from build123d import *

# Parameters (mm, degrees)
SKETCH_R          = 8.35
SKETCH_R_2        = 3.95
PAD_DEPTH         = 219
SKETCH001_R       = 1.5
POCKET_DEPTH      = 100
POCKET_DEPTH_BACK = -100


with BuildPart() as part:
    # Sketch → Pad (new body)
    with BuildSketch(Plane.XY):
        Circle(SKETCH_R)
        Circle(SKETCH_R_2, mode=Mode.SUBTRACT)
    extrude(amount=PAD_DEPTH)

    # Sketch001 → Pocket (cut, two sides)
    with BuildSketch(Plane.XZ) as pocket_sk:
        with Locations((0, 109.5)):
            Circle(SKETCH001_R)
        with Locations((0, 189)):
            Circle(SKETCH001_R)
        with Locations((0, 30)):
            Circle(SKETCH001_R)
    extrude(amount=-POCKET_DEPTH, mode=Mode.SUBTRACT)
    extrude(pocket_sk.sketch, amount=-POCKET_DEPTH_BACK, mode=Mode.SUBTRACT)


solid = part.part
For this review, take the finished solid that the model builds, in its own axes (mm). Give positions to 0.01 mm unless a question says otherwise; leave off trailing zeros. Order: outer loops, then holes, each group sorted by start corner. A loop starts at its lowest first (then second) coordinate and runs counter-clockwise, first axis right, second up. Notation, with made-up numbers: (73.5, 39.5) - (90.5, 39.5) arc R15 ccw to (90.5, 64.5) - close; hole circle Ø4 at (-13.75, -23). An arc over 180 degrees is marked (long way). Answer as a JSON object with one key per item and string values. Group by question number.
Item 1: Take a section at A-A on y = 0. Give the boundary of the cut face in (x, z), and give its area (3 significant figures).
Item 2: Take a section at C-C on x = -6. Give the boundary of the cut face in (y, z).
Item 3: Wall thickness on line 1 along Z through (x, y) = (0, -6.35); line 2 along Z through (x, y) = (1, -5.25); line 3 along Y through (x, z) = (-1, 147): over which ranges is each line inside the solid? List them lowest first.
Item 4: Clearance check with flat-ended pins moving along their axes: pin 1 Ø1 at (x, z) = (-1.5, 77.5) entering from -Y; pin 2 Ø6 at (y, z) = (-6.5, 49.5) entering from -X; pin 3 Ø1 at (y, z) = (-6.5, 31.5) entering from +X. State where each tip first meets the part, or that it passes through.
Item 5: Draft analysis for pull direction X (two halves, no side actions). For faces 1 (the cylindrical face through (7.964, 2.508, 107.967)), 2 (the cylindrical face through (-3.135, -2.404, 107.967)), 3 (the flat face through (4, -2, 219)), state which applies: pulls with the +X half, pulls with the -X half, needs draft (parallel to the pull), parting line crosses it, or undercut.
Item 6: Take a section at B-B on z = 145. Give the boundary of the cut face in (x, y).
Reported:
{
 "1": {"outline": "(-8.35, 0) - (-3.95, 0) - (-3.95, 219) - (-8.35, 219) - close; (3.95, 0) - (8.35, 0) - (8.35, 219) - (3.95, 219) - close", "area": "1,930 mm^2"},
 "2": {"outline": "(-5.81, 0) - (5.81, 0) - (5.81, 219) - (-5.81, 219) - close"},
 "3": {"line 1": "0 to 28.5, 31.5 to 108, 111 to 187.5, 190.5 to 219", "line 2": "0 to 28.88, 31.12 to 108.38, 110.62 to 187.88, 190.12 to 219", "line 3": "-8.29 to -3.82, 3.82 to 8.29"},
 "4": {"pin 1": "y = -8.29", "pin 2": "x = -7.58", "pin 3": "x = 5.81"},
 "5": {"face 1": "parting line crosses it", "face 2": "undercut", "face 3": "needs draft"},
 "6": {"outline": "circle Ø16.7 at (0, 0); hole circle Ø7.9 at (0, 0)"}
}
